from build123d import *

# Parameters (mm, degrees)
SKETCH1_W                                        = 35
SKETCH1_H                                        = 32.5
BOSS_EXTRUDE1_DEPTH                              = 14
CBORE_FOR_1_4_SOCKET_HEAD_CAP_SCREW1_D           = 6.7564
CBORE_FOR_1_4_SOCKET_HEAD_CAP_SCREW1_CBORE_D     = 11.1125
CBORE_FOR_1_4_SOCKET_HEAD_CAP_SCREW1_CBORE_DEPTH = 6.35
SKETCH18_R                                       = 1.2065
SPRING_END_HOLE_DEPTH                            = 40.477841886
SKETCH19_W                                       = 17
SKETCH19_H                                       = 32.5
BOSS_EXTRUDE2_DEPTH                              = 14
CBORE_FOR_1_4_SOCKET_HEAD_CAP_SCREW2_D           = 6.7564
CBORE_FOR_1_4_SOCKET_HEAD_CAP_SCREW2_CBORE_D     = 11.1125
CBORE_FOR_1_4_SOCKET_HEAD_CAP_SCREW2_CBORE_DEPTH = 6.35
SKETCH22_R                                       = 2.0828
CUT_EXTRUDE1_DEPTH                               = 10


with BuildPart() as part:
    # Sketch1 → Boss-Extrude1 (new body)
    with BuildSketch(Plane.XY):
        Rectangle(SKETCH1_W, SKETCH1_H)
    extrude(amount=BOSS_EXTRUDE1_DEPTH)

    # CBORE for 1/4 Socket Head Cap Screw1 (through all)
    with Locations(Plane.XY.offset(14)):
        with Locations((0, -8.5), (0, 8.5)):
            CounterBoreHole(CBORE_FOR_1_4_SOCKET_HEAD_CAP_SCREW1_D / 2, CBORE_FOR_1_4_SOCKET_HEAD_CAP_SCREW1_CBORE_D / 2, CBORE_FOR_1_4_SOCKET_HEAD_CAP_SCREW1_CBORE_DEPTH)

    # Sketch18 → Spring-End Hole (cut, through all)
    with BuildSketch(Plane(origin=(0, 16.25, 0), x_dir=(1, 0, 0), z_dir=(0, 1, 0))):
        with Locations(Location((11.9761, -9, 0), (0, 0, 270))):
            Circle(SKETCH18_R)
    extrude(amount=-SPRING_END_HOLE_DEPTH, mode=Mode.SUBTRACT)

    # Sketch19 → Boss-Extrude2 (add)
    with BuildSketch(Plane.XY.offset(14)):
        with Locations((-26, 0)):
            Rectangle(SKETCH19_W, SKETCH19_H)
    extrude(amount=-BOSS_EXTRUDE2_DEPTH)

    # CBORE for 1/4 Socket Head Cap Screw2 (through all)
    with Locations(Plane.XY.offset(14)):
        with Locations((-17, 8.5), (-17, -8.5)):
            CounterBoreHole(CBORE_FOR_1_4_SOCKET_HEAD_CAP_SCREW2_D / 2, CBORE_FOR_1_4_SOCKET_HEAD_CAP_SCREW2_CBORE_D / 2, CBORE_FOR_1_4_SOCKET_HEAD_CAP_SCREW2_CBORE_DEPTH)

    # Sketch22 → Cut-Extrude1 (cut)
    with BuildSketch(Plane.ZY.offset(34.5)):
        with Locations((7, 0.5882)):
            Circle(SKETCH22_R)
        with Locations((7, -10.4354)):
            Circle(SKETCH22_R)
    cut_extrude1 = extrude(amount=-CUT_EXTRUDE1_DEPTH, mode=Mode.SUBTRACT)

    # Mirror1: Cut-Extrude1 across plane
    add(cut_extrude1.mirror(Plane(origin=(-8.5, 0, 0), x_dir=(0, 0, 1), z_dir=(1, 0, 0))), mode=Mode.SUBTRACT)


solid = part.part
The model under review builds one solid part; all positions refer to its coordinate system, in mm. A direction names the side the tool comes from. Give positions to 0.01 mm unless a question says otherwise; leave off trailing zeros. Order: outer loops, then holes, each group sorted by start corner. A loop starts at its lowest first (then second) coordinate and runs counter-clockwise, first axis right, second up. Notation, with made-up numbers: M -11.75,77.5 L 32.25,77.5 A22 ccw 32.25,111.5 Z; hole C 10,40.5 d11. An arc over 180 degrees is marked long. One line per question, with ' | ' between items. Start each with the question number.
1) Consider section C-C, the plane z = 7. Give the boundary of the cut face in (x, y), then the cut area to 3 significant figures.
2) Consider section D-D, the plane y = -11. State how many separate pieces and enclosed holes the cut face has, then the cut area to 3 significant figures.
3) Mouldability with a two-part tool opening along Z and no side actions: class faces 5 (the face through (-29.57, -9.81, 8.987)), 6 (the face through (-18.816, 11.349, 3.771)), 7 (the face through (-9, 0, 14)) as pulls with the +Z half, pulls with the -Z half, needs draft (parallel to the pull), parting line crosses it, or undercut.
4) Consider section B-B, the plane y = 10. Give the boundary of the cut face in (x, z).
5) For faces 1 (the face through (0.44, 11.85, 3.77)), 2 (the face through (7.5, 1, 7)), 3 (the face through (-17.1, 4.9, 7.65)), 4 (the face through (-24.5, 1, 7)), list the 3-axis set-ups (+Z, -Z, +X, -X, +Y, -Y) from which the entire face can be reached by the end or side of a thin tool; tool diameter is ignored.
6) Consider section A-A, the plane x = 0. Give the boundary of the cut face in (y, z).
7) Clearance check with flat-ended pins moving along their axes: P1, Ø5.5, axis at y = 0.59, z = 7, coming from the +X side; P2, Ø3.5, axis at x = 0, y = -10.5, coming from the +Z side; P3, Ø3.5, axis at y = -10.44, z = 7, coming from the -X side. State where each tip first meets the part, or that it passes through.
8) Wall thickness on L1, parallel to Y at x = 0, z = 12.5; L2, parallel to X at y = 9, z = 13.75; L3, parallel to Y at x = -27.25, z = 7: over which ranges is each line inside the solid? List them lowest first. Write a range as from..to.
Found:
1) outline: M -34.5,-16.25 L 17.5,-16.25 L 17.5,-12.52 L 7.5,-12.52 L 7.5,-8.35 L 17.5,-8.35 L 17.5,-1.49 L 7.5,-1.49 L 7.5,2.67 L 17.5,2.67 L 17.5,16.25 L -34.5,16.25 L -34.5,2.67 L -24.5,2.67 L -24.5,-1.49 L -34.5,-1.49 L -34.5,-8.35 L -24.5,-8.35 L -24.5,-12.52 L -34.5,-12.52 Z; hole C -17,-8.5 d6.76; hole C -17,8.5 d6.76; hole C 0,-8.5 d6.76; hole C 0,8.5 d6.76 | area: 1,380 mm²
2) separate pieces: 3 | enclosed holes: 0 | area: 450 mm²
3) face 5: undercut | face 6: needs draft | face 7: pulls with the +Z half
4) outline: M -34.5,0 L -20.03,0 L -20.03,7.65 L -22.35,7.65 L -22.35,14 L -34.5,14 Z; M -13.97,0 L -3.03,0 L -3.03,7.65 L -5.35,7.65 L -5.35,14 L -11.65,14 L -11.65,7.65 L -13.97,7.65 Z; M 3.03,0 L 17.5,0 L 17.5,14 L 5.35,14 L 5.35,7.65 L 3.03,7.65 Z; hole C 11.98,9 d2.41
5) face 1: +Z, -Z | face 2: +X | face 3: +Z | face 4: -X
6) outline: M -16.25,0 L -11.88,0 L -11.88,7.65 L -14.06,7.65 L -14.06,14 L -16.25,14 Z; M -5.12,0 L 5.12,0 L 5.12,7.65 L 2.94,7.65 L 2.94,14 L -2.94,14 L -2.94,7.65 L -5.12,7.65 Z; M 11.88,0 L 16.25,0 L 16.25,14 L 14.06,14 L 14.06,7.65 L 11.88,7.65 Z
7) P1: stops at x = 17.5 | P2: stops at z = 7.65 | P3: stops at x = -24.5
8) L1: y = -16.25..-14.06, -2.94..2.94, 14.06..16.25 | L2: x = -34.5..-22.53, -11.47..-5.53, 5.53..17.5 | L3: y = -16.25..-12.52, -8.35..-1.49, 2.67..16.25
